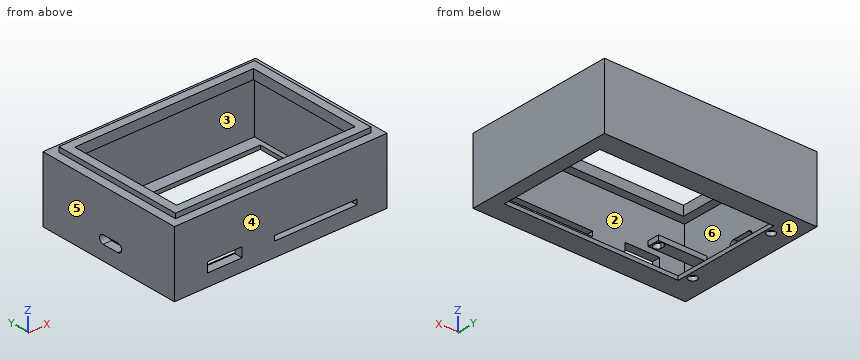
from build123d import *

# Parameters (mm, degrees)
SKETCH_1_W          = 88
SKETCH_1_H          = 62
EXTRUDE_1_DEPTH     = 2
SKETCH_2_W          = 81
SKETCH_2_H          = 55
SKETCH_2_W_2        = 74
SKETCH_2_H_2        = 48
EXTRUDE_2_DEPTH     = 2
SKETCH_3_W          = 88
SKETCH_3_H          = 62
SKETCH_3_W_2        = 81
SKETCH_3_H_2        = 55
EXTRUDE_3_DEPTH     = 25
SKETCH_5_W          = 74
SKETCH_5_H          = 48
CUT_EXTRUDE_1_DEPTH = 20
SKETCH_6_W          = 7
SKETCH_6_H          = 45
SKETCH_6_R          = 1.75
SKETCH_6_W_2        = 2
EXTRUDE_4_DEPTH     = 1.6
SKETCH_8_W          = 2
SKETCH_8_H          = 5
EXTRUDE_5_DEPTH     = 20
CUT_EXTRUDE_2_DEPTH = 17
SKETCH_7_W          = 34
SKETCH_7_H          = 2
SKETCH_7_W_2        = 14.295678294
SKETCH_7_H_2        = 4
CUT_EXTRUDE_3_DEPTH = 5
CUT_EXTRUDE_4_DEPTH = 5


with BuildPart() as part:
    # 草图1 → 凸台-拉伸1 (new body)
    with BuildSketch(Plane.XY):
        with Locations((44, -31)):
            Rectangle(SKETCH_1_W, SKETCH_1_H)
    extrude(amount=EXTRUDE_1_DEPTH)

    # 草图2 → 凸台-拉伸2 (add)
    with BuildSketch(Plane.XY.offset(2)):
        with Locations((44, -31)):
            Rectangle(SKETCH_2_W, SKETCH_2_H)
        with Locations((44, -31)):
            Rectangle(SKETCH_2_W_2, SKETCH_2_H_2, mode=Mode.SUBTRACT)
    extrude(amount=EXTRUDE_2_DEPTH)

    # 草图3 → 凸台-拉伸3 (add)
    with BuildSketch(Plane(origin=(0, 0, 0), x_dir=(-1, 0, 0), z_dir=(0, 0, -1))):
        with Locations((-44, -31)):
            Rectangle(SKETCH_3_W, SKETCH_3_H)
        with Locations((-44, -31)):
            Rectangle(SKETCH_3_W_2, SKETCH_3_H_2, mode=Mode.SUBTRACT)
    extrude(amount=EXTRUDE_3_DEPTH)

    # 草图5 → 切除-拉伸1 (cut)
    with BuildSketch(Plane.XY.offset(2)):
        with Locations((44, -31)):
            Rectangle(SKETCH_5_W, SKETCH_5_H)
    extrude(amount=-CUT_EXTRUDE_1_DEPTH, mode=Mode.SUBTRACT)

    # 草图6 → 凸台-拉伸4 (add)
    with BuildSketch(Plane(origin=(0, 0, -25), x_dir=(-1, 0, 0), z_dir=(0, 0, -1))):
        Polygon((-3.5, -3.5), (-84.5, -3.5), (-84.5, -8.5), (-82.5, -8.5), (-10.5, -8.5), (-3.5, -8.5), align=None)
        with Locations((-7, -31)):
            Rectangle(SKETCH_6_W, SKETCH_6_H)
        with Locations((-8, -49.5)):
            Circle(SKETCH_6_R, mode=Mode.SUBTRACT)
        with Locations((-8, -12.5)):
            Circle(SKETCH_6_R, mode=Mode.SUBTRACT)
        with Locations((-83.5, -31)):
            Rectangle(SKETCH_6_W_2, SKETCH_6_H)
        Polygon((-82.5, -53.5), (-84.5, -53.5), (-84.5, -58.5), (-3.5, -58.5), (-3.5, -53.5), (-10.5, -53.5), align=None)
    extrude(amount=-EXTRUDE_4_DEPTH)

    # 草图8 → 凸台-拉伸5 (add)
    with BuildSketch(Plane(origin=(3.5, 0, 0), x_dir=(0, 0, -1), z_dir=(1, 0, 0))):
        with Locations((17, -50.5)):
            Rectangle(SKETCH_8_W, SKETCH_8_H)
    extrude(amount=EXTRUDE_5_DEPTH)

    # 草图10 → 切除-拉伸2 (cut)
    with BuildSketch(Plane(origin=(0, 0, -18), x_dir=(-1, 0, 0), z_dir=(0, 0, -1))):
        with BuildLine():
            Line((-19.62339277, -49.845001647), (-19.62339277, -51.119762416))
            ThreePointArc((-19.62339277, -51.119762416), (-21.228647072, -52.725016718), (-22.833901374, -51.119762416))
            Line((-22.833901374, -51.119762416), (-22.833901374, -49.845001647))
            ThreePointArc((-22.833901374, -49.845001647), (-21.228647072, -48.239747346), (-19.62339277, -49.845001647))
        make_face()
    extrude(amount=-CUT_EXTRUDE_2_DEPTH, mode=Mode.SUBTRACT)

    # 草图7 → 切除-拉伸3 (cut)
    with BuildSketch(Plane.XZ.offset(62)):
        with Locations((58.5, -18)):
            Rectangle(SKETCH_7_W, SKETCH_7_H)
        with Locations((20.909824804, -17.875130222)):
            Rectangle(SKETCH_7_W_2, SKETCH_7_H_2)
    extrude(amount=-CUT_EXTRUDE_3_DEPTH, mode=Mode.SUBTRACT)

    # 草图11 → 切除-拉伸4 (cut)
    with BuildSketch(Plane.ZY):
        with BuildLine():
            Line((-15.507327091, -28.393704354), (-15.507327091, -35.287349512))
            ThreePointArc((-15.507327091, -35.287349512), (-17.230738381, -37.010760802), (-18.954149671, -35.287349512))
            Line((-18.954149671, -35.287349512), (-18.954149671, -28.393704354))
            ThreePointArc((-18.954149671, -28.393704354), (-17.230738381, -26.670293064), (-15.507327091, -28.393704354))
        make_face()
    extrude(amount=-CUT_EXTRUDE_4_DEPTH, mode=Mode.SUBTRACT)


solid = part.part
CAD build for the part. Positions are in the model's coordinates, mm. Face numbers are marked on the shaded views. A direction names the side the tool comes from. Coordinates: 2 decimals unless noted, no trailing zeros. Order: outer loops, then holes, each group sorted by start corner. A loop starts at its lowest first (then second) coordinate and runs counter-clockwise, first axis right, second up. Notation, with made-up numbers: (15.5, -32.75) -> (70.5, -32.75) arc R25 ccw to (70.5, -19.75) -> close; hole circle Ø11 at (52, -36.75). An arc over 180 degrees is marked (long way). Answer in a Markdown table with one row per item.
1) Band-saw the part on B-B (x = 73.5). List the corners of the cut face in (y, z), and give its area (3 significant figures).
Check values:
| item | result |
|---|---|
| outline | (-62, -25) -> (-53.5, -25) -> (-53.5, -23.4) -> (-58.5, -23.4) -> (-58.5, -19) -> (-62, -19) -> close; (-62, -17) -> (-58.5, -17) -> (-58.5, 0) -> (-55, 0) -> (-55, 4) -> (-58.5, 4) -> (-58.5, 2) -> (-62, 2) -> close; (-8.5, -25) -> (0, -25) -> (0, 2) -> (-3.5, 2) -> (-3.5, 4) -> (-7, 4) -> (-7, 0) -> (-3.5, 0) -> (-3.5, -23.4) -> (-8.5, -23.4) -> close |
| area | 226 mm2 |
2) Mould opens along X. For the marked faces 3, 4, 5 and 6 say: pulls with the +X half, pulls with the -X half, needs draft (parallel to the pull), parting line crosses it, or undercut.
Check values:
| item | result |
|---|---|
| face 3 | undercut |
| face 4 | needs draft |
| face 5 | pulls with the -X half |
| face 6 | undercut |
3) Which spindle directions (+Z, -Z, +X, -X, +Y, -Y) get a long thin tool onto all of the face, cutting with end or side? Do the marked faces 1 and 2. Say none if no direction does.
Check values:
| item | result |
|---|---|
| face 1 | -Z, +X, -X, +Y, -Y |
| face 2 | none |
4) Flat gauge pins, fed straight in: P1, Ø6, axis at x = 18, y = -45.5, coming from the +Z side; P2, Ø4, axis at x = 1, y = -33, coming from the +Z side. Where does each tip first touch, or does it go through?
Check values:
| item | result |
|---|---|
| P1 | z = -16 |
| P2 | z = 2 |
5) Band-saw the part on A-A (x = 8). List the corners of the cut face in (y, z), and give its area (3 significant figures).
Check values:
| item | result |
|---|---|
| outline | (-62, -25) -> (-51.25, -25) -> (-51.25, -23.4) -> (-58.5, -23.4) -> (-58.5, 0) -> (-55, 0) -> (-55, 4) -> (-58.5, 4) -> (-58.5, 2) -> (-62, 2) -> close; (-53, -18) -> (-48, -18) -> (-48, -16) -> (-53, -16) -> close; (-47.75, -25) -> (-14.25, -25) -> (-14.25, -23.4) -> (-47.75, -23.4) -> close; (-10.75, -25) -> (0, -25) -> (0, 2) -> (-3.5, 2) -> (-3.5, 4) -> (-7, 4) -> (-7, 0) -> (-3.5, 0) -> (-3.5, -23.4) -> (-10.75, -23.4) -> close |
| area | 304 mm2 |
6) Drill centre lines: line 1 (Y direction, x = 8, z = -23.85); line 2 (Y direction, x = 7, z = -22.5); line 3 (X direction, y = -27.5, z = -7). Where is each one in solid material? Low to high.
Check values:
| item | result |
|---|---|
| line 1 | -62 to -51.25, -47.75 to -14.25, -10.75 to 0 |
| line 2 | -62 to -58.5, -3.5 to 0 |
| line 3 | 0 to 3.5, 84.5 to 88 |
7) Band-saw the part on C-C (y = -12.5). List the corners of the cut face in (x, z), and give its area (3 significant figures).
Check values:
| item | result |
|---|---|
| outline | (0, -25) -> (6.25, -25) -> (6.25, -23.4) -> (3.5, -23.4) -> (3.5, 0) -> (7, 0) -> (7, 4) -> (3.5, 4) -> (3.5, 2) -> (0, 2) -> close; (9.75, -25) -> (10.5, -25) -> (10.5, -23.4) -> (9.75, -23.4) -> close; (81, 0) -> (84.5, 0) -> (84.5, -23.4) -> (82.5, -23.4) -> (82.5, -25) -> (88, -25) -> (88, 2) -> (84.5, 2) -> (84.5, 4) -> (81, 4) -> close |
| area | 226 mm2 |
8) Band-saw the part on D-D (z = -6.75). List the corners of the cut face in (x, y), and give its area (3 significant figures).
Check values:
| item | result |
|---|---|
| outline | (0, -62) -> (88, -62) -> (88, 0) -> (0, 0) -> close; hole (3.5, -58.5) -> (84.5, -58.5) -> (84.5, -3.5) -> (3.5, -3.5) -> close |
| area | 1,000 mm2 |
